```python
from build123d import *

# Parameters (mm, degrees)
BOSS_EXTRUDE1_DEPTH = 1
SKETCH2_R           = 3.175
CUT_EXTRUDE1_DEPTH  = 2
CUT_EXTRUDE2_DEPTH  = 2


with BuildPart() as part:
    # Sketch1 → Boss-Extrude1 (new body)
    with BuildSketch(Plane.XY):
        with BuildLine():
            Line((10.237514752, 28.034216891), (15.100684157, 39.774946424))
            ThreePointArc((15.100684157, 39.774946424), (-16.28126663, -39.306454711), (17.447338169, 38.802930505))
            Line((17.447338169, 38.802930505), (12.097700571, 25.88776286))
            ThreePointArc((12.097700571, 25.88776286), (-21.083635895, -19.287584671), (26.859778778, 9.751046558))
            Line((26.859778778, 9.751046558), (15.105587123, 4.88230096))
            ThreePointArc((15.105587123, 4.88230096), (-14.666587579, -6.075099489), (14.133571205, 7.228954972))
            Line((14.133571205, 7.228954972), (27.062200973, 12.584168765))
            ThreePointArc((27.062200973, 12.584168765), (-20.186460687, -21.982511911), (10.237514752, 28.034216891))
        make_face()
    extrude(amount=BOSS_EXTRUDE1_DEPTH)

    # Sketch2 → Cut-Extrude1 (cut, through all)
    with BuildSketch(Plane.XY.offset(1)):
        with Locations((22.225, 1.106e-06)):
            Circle(SKETCH2_R)
        with Locations((36.195, 0)):
            Circle(SKETCH2_R)
        with Locations((15.715448994, -15.71544743)):
            Circle(SKETCH2_R)
        with Locations((25.593729945, -25.593729945)):
            Circle(SKETCH2_R)
        with Locations((1.106e-06, -22.225)):
            Circle(SKETCH2_R)
        with Locations((0, -36.195)):
            Circle(SKETCH2_R)
        with Locations((-15.71544743, -15.715448994)):
            Circle(SKETCH2_R)
        with Locations((-25.593729945, -25.593729945)):
            Circle(SKETCH2_R)
        with Locations((-22.225, -1.106e-06)):
            Circle(SKETCH2_R)
        with Locations((-36.195, 0)):
            Circle(SKETCH2_R)
        with Locations((-15.715448994, 15.71544743)):
            Circle(SKETCH2_R)
        with Locations((-25.593729945, 25.593729945)):
            Circle(SKETCH2_R)
        with Locations((-1.106e-06, 22.225)):
            Circle(SKETCH2_R)
        with Locations((0, 36.195)):
            Circle(SKETCH2_R)
        with Locations((15.71544743, 15.715448994)):
            Circle(SKETCH2_R)
        with Locations((25.593729945, 25.593729945)):
            Circle(SKETCH2_R)
    extrude(amount=-CUT_EXTRUDE1_DEPTH, mode=Mode.SUBTRACT)

    # Sketch3 → Cut-Extrude2 (cut, through all)
    with BuildSketch(Plane.XY.offset(1)):
        Polygon((25.327186179, -11.865502107), (26.500513186, -12.351510066), (27.472529104, -10.004856053), (26.299202097, -9.518848094), align=None)
        Polygon((10.004856053, -27.472529104), (12.351510066, -26.500513186), (11.865502107, -25.327186179), (9.518848094, -26.299202097), align=None)
        Polygon((-12.351510066, -26.500513186), (-10.004856053, -27.472529104), (-9.518848094, -26.299202097), (-11.865502107, -25.327186179), align=None)
        Polygon((-27.472529104, -10.004856053), (-26.500513186, -12.351510066), (-25.327186179, -11.865502107), (-26.299202097, -9.518848094), align=None)
        Polygon((-26.500513186, 12.351510066), (-27.472529104, 10.004856053), (-26.299202097, 9.518848094), (-25.327186179, 11.865502107), align=None)
        Polygon((-10.004856053, 27.472529104), (-12.351510066, 26.500513186), (-11.865502107, 25.327186179), (-9.518848094, 26.299202097), align=None)
        Polygon((12.351510066, 26.500513186), (10.004856053, 27.472529104), (9.518848094, 26.299202097), (11.865502107, 25.327186179), align=None)
        Polygon((39.205799167, 14.864935644), (40.379126173, 15.350943603), (39.407110255, 17.697597616), (38.233783248, 17.211589657), align=None)
        Polygon((39.205799167, -14.864935644), (40.379126173, -15.350943603), (39.407110255, -17.697597616), (38.233783248, -17.211589657), align=None)
        Polygon((17.211589657, -38.233783248), (17.697597616, -39.407110255), (15.350943603, -40.379126173), (14.864935644, -39.205799167), align=None)
        Polygon((-14.864935644, -39.205799167), (-15.350943603, -40.379126173), (-17.697597616, -39.407110255), (-17.211589657, -38.233783248), align=None)
        Polygon((-38.233783248, -17.211589657), (-39.407110255, -17.697597616), (-40.379126173, -15.350943603), (-39.205799167, -14.864935644), align=None)
        Polygon((-39.205799167, 14.864935644), (-40.379126173, 15.350943603), (-39.407110255, 17.697597616), (-38.233783248, 17.211589657), align=None)
        Polygon((-17.211589657, 38.233783248), (-17.697597616, 39.407110255), (-15.350943603, 40.379126173), (-14.864935644, 39.205799167), align=None)
    extrude(amount=-CUT_EXTRUDE2_DEPTH, mode=Mode.SUBTRACT)


solid = part.part
```
Work out the finished part from the listing and answer in its coordinate system (mm). A direction names the side the tool comes from. Round coordinates to 2 decimals unless told otherwise and drop trailing zeros.
1) A flat-ended cylindrical pin translates along its axis: P1, Ø5, axis at x = 15.72, y = 15.72, coming from the +Z side. Find the tip coordinate at first contact, or state that the pin passes through.
2) Consider probe 1 along X at (y, z) = (25.5, 0.8); probe 2 along Y at (x, z) = (-16, 0.9); probe 3 along Y at (x, z) = (17, 0.95). Determine where each line is inside the solid, lowest interval first.
3) A cutting plane is placed at A-A on x = 0. Give the number of separate pieces and of enclosed holes in the cut face, and give its area (3 significant figures).
4) Determine the mould class of faces 1 (the face through (21.06, 7.35, 0.49)), 2 (the face through (-30.236, -29.931, 0.493)), 3 (the face through (42.544, -0.216, 0.493)) for opening direction Y: pulls with the +Y half, pulls with the -Y half, needs draft (parallel to the pull), parting line crosses it, or undercut.
5) Which of the six approach directions +Z, -Z, +X, -X, +Y, -Y give full straight-line access (tool end or side, diameter ignored) to faces 4 (the face through (12.635, 33.822, 0.493)), 5 (the face through (-1, -18, 1))?
Entries:
1. P1: passes through
2. probe 1: x = -34.06 to -28.77, -22.42 to -15.51, -12.89 to -11.94, -11.45 to 11.45, 11.94 to 22.42, 28.77 to 34.06
2. probe 2: y = -38.74 to -25.19, -23.68 to -18.88, -12.55 to 12.55, 18.88 to 23.68, 25.19 to 38.74
2. probe 3: y = -38.32 to -24.53, -22.97 to -18.62, -12.81 to 5.67, 8.42 to 12.81, 18.62 to 37.72
3. separate pieces: 8
3. enclosed holes: 0
3. area: 25.4 mm2
4. face 1: undercut
4. face 2: pulls with the -Y half
4. face 3: parting line crosses it
5. face 4: +Z, -Z
5. face 5: +Z, +X, -X, +Y, -Y
